```python
from build123d import *

# Parameters (mm, degrees)
SKETCH1_R               = 50
BOSS_EXTRUDE1_DEPTH     = 10
BOSS_EXTRUDE2_DEPTH     = 40
CUT_EXTRUDE1_DEPTH      = 10
CUT_EXTRUDE1_DEPTH_BACK = 51
SKETCH3_R               = 5
CUT_EXTRUDE3_DEPTH      = 51
CUT_EXTRUDE3_DEPTH_BACK = 51


with BuildPart() as part:
    # Sketch1 → Boss-Extrude1 (new body)
    with BuildSketch(Plane.XY):
        Circle(SKETCH1_R)
    extrude(amount=BOSS_EXTRUDE1_DEPTH)

    # Sketch2 → Boss-Extrude2 (add)
    with BuildSketch(Plane.XY.offset(10)):
        Polygon((0, 15), (20, 15), (20, 25), (0, 25), (-20, 25), (-20, 15), align=None)
        Polygon((0, -15), (20, -15), (20, -25), (0, -25), (-20, -25), (-20, -15), align=None)
    extrude(amount=BOSS_EXTRUDE2_DEPTH)

    # Sketch3 → Cut-Extrude1 (cut, two sides: drawn at the far end of the back side and taken through both)
    with BuildSketch(Plane(origin=(0, 25, 0), x_dir=(1, 0, 0), z_dir=(0, 1, 0)).offset(-CUT_EXTRUDE1_DEPTH_BACK)):
        with Locations(Location((0, -30, 0), (0, 0, 90))):
            Circle(SKETCH3_R)
    extrude(amount=CUT_EXTRUDE1_DEPTH + CUT_EXTRUDE1_DEPTH_BACK, mode=Mode.SUBTRACT)

    # Sketch4 → Cut-Extrude3 (cut, two sides: drawn at the far end of the back side and taken through both)
    with BuildSketch(Plane.XZ.offset(25).offset(-CUT_EXTRUDE3_DEPTH_BACK)):
        with BuildLine():
            Line((-20, 30), (-47.366486711, 30))
            Line((-47.366486711, 30), (-38.964183934, 74.74544014))
            Line((-38.964183934, 74.74544014), (40.839267743, 70.572196031))
            Line((40.839267743, 70.572196031), (55.137019974, 30))
            Line((55.137019974, 30), (20, 30))
            ThreePointArc((20, 30), (0, 50), (-20, 30))
        make_face()
    extrude(amount=CUT_EXTRUDE3_DEPTH + CUT_EXTRUDE3_DEPTH_BACK, mode=Mode.SUBTRACT)


solid = part.part
```
Read the model definition and answer for the solid it produces. Units are mm, in the model's axes. A direction names the side the tool comes from. Coordinates: 2 decimals unless noted, no trailing zeros. Write each loop counter-clockwise with the first axis right and the second up, starting at its lowest first coordinate (ties: lowest second). Pieces come first, ordered by that corner, then holes. Notation, with made-up numbers: (5, -5) -> (41, -5) arc R29 ccw to (41, 27) -> close; hole circle Ø3 at (-25.75, 74). An arc over 180 degrees is marked (long way). Write item = value, one per line.
(1) Section B-B on x = 0 is taken. Write down the section's boundary in (y, z).
From the geometry:
outline = (-50, 0) -> (50, 0) -> (50, 10) -> (25, 10) -> (25, 25) -> (15, 25) -> (15, 10) -> (-15, 10) -> (-15, 25) -> (-25, 25) -> (-25, 10) -> (-50, 10) -> close; (-25, 35) -> (-15, 35) -> (-15, 50) -> (-25, 50) -> close; (15, 35) -> (25, 35) -> (25, 50) -> (15, 50) -> close
(2) Section D-D on y = 0 is taken. Write down the section's boundary in (x, z), plus the area to 3 significant figures.
From the geometry:
outline = (-50, 0) -> (50, 0) -> (50, 10) -> (-50, 10) -> close
area = 1,000 mm2
(3) Given pin 1 Ø8 at (y, z) = (-18.5, 21) entering from -X; pin 2 Ø3 at (y, z) = (22, 23) entering from +X; pin 3 Ø12 at (x, z) = (-9, 36.5) entering from -Y, each flat-ended and moving along its own axis, determine where each tip first touches the part or whether it passes through.
From the geometry:
pin_1 = -20
pin_2 = 20
pin_3 = -25
(4) Straight lines are drawn through the part: L1, parallel to X at y = -20, z = 30; L2, parallel to Y at x = 9.5, z = 33; L3, parallel to Z at x = -21.5, y = 10. For each, find the intervals that lie inside material, in ascending order. Write a range as from..to.
From the geometry:
L1 = -20..-5, 5..20
L2 = -25..-15, 15..25
L3 = 0..10
(5) Section C-C on z = 32 is taken. Write down the section's boundary in (x, y), plus the area to 3 significant figures.
From the geometry:
outline = (-19.9, -25) -> (-4.58, -25) -> (-4.58, -15) -> (-19.9, -15) -> close; (-19.9, 15) -> (-4.58, 15) -> (-4.58, 25) -> (-19.9, 25) -> close; (4.58, -25) -> (19.9, -25) -> (19.9, -15) -> (4.58, -15) -> close; (4.58, 15) -> (19.9, 15) -> (19.9, 25) -> (4.58, 25) -> close
area = 613 mm2
(6) Section A-A on z = 21 is taken. Write down the section's boundary in (x, y), plus the area to 3 significant figures.
From the geometry:
outline = (-20, -25) -> (20, -25) -> (20, -15) -> (-20, -15) -> close; (-20, 15) -> (20, 15) -> (20, 25) -> (-20, 25) -> close
area = 800 mm2
(7) Which of the six approach directions +Z, -Z, +X, -X, +Y, -Y give full straight-line access (tool end or side, diameter ignored) to faces 1 (the face through (4, 15, 25)), 2 (the face through (20, -20, 20)), 3 (the face through (4, -25, 25)), 4 (the face through (-20, -20, 20))?
From the geometry:
face_1 = +Z, +X, -X
face_2 = +Z, +X, +Y, -Y
face_3 = +Z, +X, -X, -Y
face_4 = +Z, -X, +Y, -Y
(8) For a pull along X with two mould halves and no side action, classify faces 5 (the face through (0, -20, 35)), 6 (the face through (0, 20, 50)), 7 (the face through (-1, 1, 10)) as +X half, -X half, draft (parallel to the pull), parting line (faces both ways), or undercut.
From the geometry:
face_5 = undercut
face_6 = parting line
face_7 = draft
